Geometry: final body of the model. Coordinates: model frame, mm. A direction names the side the tool comes from. Give positions to 0.01 mm unless a question says otherwise; leave off trailing zeros. Loops run counter-clockwise (first coordinate to the right, second up) from the corner with the lowest first, then second, coordinate; pieces in that order, holes last. Notation, with made-up numbers: M 80.25,21.5 L 122.25,21.5 A32 cw 122.25,55.5 Z; hole C 69.25,39 d11. An arc over 180 degrees is marked long. Put each result on its own line as item: value.
Autodesk Inventor part; units mm, degrees
ref_plane "YZ Plane" through (0, 0, 0) normal (1, 0, 0) x (0, 1, 0)
ref_plane "XZ Plane" through (0, 0, 0) normal (0, 1, 0) x (-1, 0, 0)
ref_plane "XY Plane" through (0, 0, 0) normal (0, 0, 1) x (1, 0, 0)
sketch "スケッチ1" plane through (0, 0, 0) normal (1, 0, 0) x (0, 1, 0)
  circle A0 centre (0, 0) radius 5.05
  line L0 (-10.75, 0) -> (10.75, 0) construction
  line L1 (0, 11.25) -> (0, -41) construction
  line L2 (-10.75, 0) -> (-10.75, -36)
  line L3 (-10.75, -36) -> (-10.75, -41)
  line L4 (-10.75, -41) -> (10.75, -41)
  circle A1 centre (0, 8.5) radius 1.35
  circle A2 centre (0, 8.5) radius 2.25 construction
  circle A3 centre (-8.5, 0) radius 1.35
  circle A4 centre (0, -8.5) radius 1.35
  circle A5 centre (8.5, 0) radius 1.35
  line L5 (3.75, -36) -> (-3.75, -36) construction
  line L6 (-3.75, -36) -> (-3.75, -38.5) construction
  line L7 (-3.75, -38.5) -> (3.75, -38.5) construction
  line L8 (3.75, -38.5) -> (3.75, -36) construction
  line L9 (3.75, -36) -> (-3.75, -38.5) construction
  line L10 (-3.75, -36) -> (3.75, -38.5) construction
  circle A6 centre (-7.75, -38) radius 1.6
  line L11 (-10.75, -38) -> (13.8581, -38) construction
  circle A7 centre (-7.75, -38) radius 2.75 construction
  line L12 (-3.8, -35.95) -> (3.8, -35.95)
  line L13 (3.8, -35.95) -> (3.8, -38.55)
  line L14 (3.8, -38.55) -> (-3.8, -38.55)
  line L15 (-3.8, -38.55) -> (-3.8, -35.95)
  line L16 (-3.8, -35.95) -> (3.8, -38.55) construction
  line L17 (3.8, -35.95) -> (-3.8, -38.55) construction
  arc A8 (-1.7, -35.95) -> (-3.8, -35.95) centre (-2.75, -35.95) ccw
  line L18 (-3.75, -37.25) -> (3.75, -37.25) construction
  arc A9 (-3.8, -38.55) -> (-1.7, -38.55) centre (-2.75, -38.55) ccw
  line L19 (10.75, 0) -> (10.75, -36)
  line L20 (10.75, -36) -> (10.75, -41)
  circle A10 centre (7.75, -38) radius 1.6
  circle A11 centre (7.75, -38) radius 2.75 construction
  arc A12 (3.8, -35.95) -> (1.7, -35.95) centre (2.75, -35.95) ccw
  arc A13 (1.7, -38.55) -> (3.8, -38.55) centre (2.75, -38.55) ccw
  arc A14 (10.75, 0) -> (-10.75, 0) centre (0, 0) ccw
  line L21 (-13.5, 1) -> (13.5, 1) construction
  circle A15 centre (-13.5, 1) radius 2.25 construction
  point P0 (0, -37.25)
  point P1 (1.7, -38.55)
  point P2 (-1.7, -38.55)
  point P3 (0, 1)
  dimension "d0" = 10.1
  dimension "d1" = 5
  dimension "d2" = 41
  dimension "d4" = 2.7
  dimension "d5" = 8.5
  dimension "d6" = 4.5
  dimension "d9" = 360
  dimension "d11" = 7.5
  dimension "d12" = 2.5
  dimension "d13" = 3.2
  dimension "d14" = 5.5
  dimension "d15" = 3
  dimension "d16" = 0.05
  dimension "d17" = 0.05
  dimension "d18" = 1.05
  dimension "d19" = 15.5
  dimension "d22" = 27
  dimension "d23" = 1
  dimension "d25" = 4.5
  dimension "d26" = 21.5
extrude "押し出し1" add sketch "スケッチ1" along normal blind 3
equation "\"d17\" = d16"
properties part number "Foot_back_frame" material "アルミニウム 2014-T4"
Item 1: Pin query (flat end, axial travel): pin 1 Ø1.6 at (y, z) = (-8.5, 0) entering from +X. Return the tip coordinate at first contact, or that it passes through.
Output values:
pin 1: through
Item 2: Section A-A on x = 2.2. Count the separate pieces of the cut face and the enclosed holes in it, then the cut area to 3 significant figures.
Output values:
separate pieces: 1
enclosed holes: 8
area: 917 mm²
Item 3: Mould query, pull axis Y, two halves, no side actions, for faces 1 (the cylindrical face through (1.479, -7.212, -0.406)), 2 (the cylindrical face through (1.479, -0.236, 10.747)), 3 (the flat face through (1, -10.75, -20)), 4 (the flat face through (1, 0, -41)). Classes: pulls with the +Y half, pulls with the -Y half, needs draft (parallel to the pull), parting line crosses it, or undercut.
Output values:
face 1: undercut
face 2: parting line crosses it
face 3: pulls with the -Y half
face 4: needs draft
Item 4: Set-up query: faces 5 (the flat face through (1, 0, -35.95)), 6 (the flat face through (1, 10.75, -20)). Return all of +Z, -Z, +X, -X, +Y, -Y with unobstructed straight access to the full face (end or side cutting, diameter ignored); none if empty.
Output values:
face 5: +X, -X
face 6: +Z, -Z, +X, -X, +Y
Item 5: Section D-D on y = 4.25. Output: boundary loops of the cut face in (x, z), then the cut area to 3 significant figures.
Output values:
outline: M 0,-41 L 3,-41 L 3,-2.73 L 0,-2.73 Z; M 0,2.73 L 3,2.73 L 3,9.87 L 0,9.87 Z
area: 136 mm²
Item 6: Section B-B on y = 7.75. Output: boundary loops of the cut face in (x, z).
Output values:
outline: M 0,-41 L 3,-41 L 3,-39.6 L 0,-39.6 Z; M 0,-36.4 L 3,-36.4 L 3,-1.12 L 0,-1.12 Z; M 0,1.12 L 3,1.12 L 3,7.45 L 0,7.45 Z
Item 7: Section C-C on z = -2. Output: boundary loops of the cut face in (x, y), then the cut area to 3 significant figures.
Output values:
outline: M 0,-10.75 L 3,-10.75 L 3,-4.64 L 0,-4.64 Z; M 0,4.64 L 3,4.64 L 3,10.75 L 0,10.75 Z
area: 36.7 mm²
Item 8: Line query: probe 1 along Z at (x, y) = (1.5, 0); probe 2 along Z at (x, y) = (0.8, 7.75); probe 3 along Z at (x, y) = (0.8, 3.5). Output: solid intervals per line, ascending. Write a range as [from, to].
Output values:
probe 1: [-41, -38.55], [-35.95, -9.85], [-7.15, -5.05], [5.05, 7.15], [9.85, 10.75]
probe 2: [-41, -39.6], [-36.4, -1.12], [1.12, 7.45]
probe 3: [-41, -39.28], [-35.22, -3.64], [3.64, 10.16]
